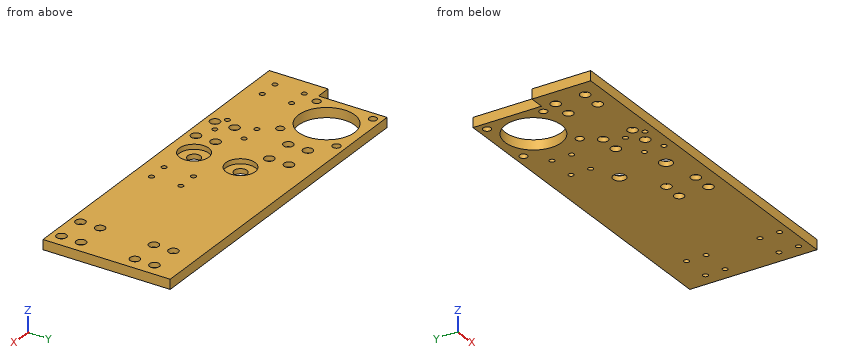
from build123d import *

# Parameters (mm, degrees)
SKETCH_1_R          = 11.5
SKETCH_1_R_2        = 1.6
SKETCH_1_R_3        = 1.05
SKETCH_1_R_4        = 2.6
EXTRUDE_1_DEPTH     = 4
SKETCH_2_R          = 2
SKETCH_2_R_2        = 6
CUT_EXTRUDE_1_DEPTH = 2
SKETCH_5_R          = 2
CUT_EXTRUDE_2_DEPTH = 2


with BuildPart() as part:
    # 草图1 → 凸台-拉伸1 (new body)
    with BuildSketch(Plane.XY):
        Polygon((0, 0), (135, 0), (135, -52), (0, -52), (-8, -52), (-8, -28), (-2, -28), (-2, 0), align=None)
        with Locations((13, -15)):
            Circle(SKETCH_1_R, mode=Mode.SUBTRACT)
        with Locations((1.5, -3.5)):
            Circle(SKETCH_1_R_2, mode=Mode.SUBTRACT)
        with Locations((24.5, -3.5)):
            Circle(SKETCH_1_R_2, mode=Mode.SUBTRACT)
        with Locations((1.5, -26.5)):
            Circle(SKETCH_1_R_2, mode=Mode.SUBTRACT)
        with Locations((24.5, -26.5)):
            Circle(SKETCH_1_R_2, mode=Mode.SUBTRACT)
        with Locations((32.5, -10)):
            Circle(SKETCH_1_R_3, mode=Mode.SUBTRACT)
        with Locations((44.5, -10)):
            Circle(SKETCH_1_R_3, mode=Mode.SUBTRACT)
        with Locations((32.5, -18)):
            Circle(SKETCH_1_R_3, mode=Mode.SUBTRACT)
        with Locations((44.5, -18)):
            Circle(SKETCH_1_R_3, mode=Mode.SUBTRACT)
        with Locations((117.5, -10)):
            Circle(SKETCH_1_R_3, mode=Mode.SUBTRACT)
        with Locations((129.5, -10)):
            Circle(SKETCH_1_R_3, mode=Mode.SUBTRACT)
        with Locations((117.5, -18)):
            Circle(SKETCH_1_R_3, mode=Mode.SUBTRACT)
        with Locations((129.5, -18)):
            Circle(SKETCH_1_R_3, mode=Mode.SUBTRACT)
        with Locations((-0.75, -33)):
            Circle(SKETCH_1_R_3, mode=Mode.SUBTRACT)
        with Locations((7.25, -33)):
            Circle(SKETCH_1_R_3, mode=Mode.SUBTRACT)
        with Locations((-0.75, -45)):
            Circle(SKETCH_1_R_3, mode=Mode.SUBTRACT)
        with Locations((7.25, -45)):
            Circle(SKETCH_1_R_3, mode=Mode.SUBTRACT)
        with Locations((29.25, -33)):
            Circle(SKETCH_1_R_3, mode=Mode.SUBTRACT)
        with Locations((37.25, -33)):
            Circle(SKETCH_1_R_3, mode=Mode.SUBTRACT)
        with Locations((37.25, -45)):
            Circle(SKETCH_1_R_3, mode=Mode.SUBTRACT)
        with Locations((29.25, -45)):
            Circle(SKETCH_1_R_3, mode=Mode.SUBTRACT)
        with Locations((32.5, -40)):
            Circle(SKETCH_1_R_3, mode=Mode.SUBTRACT)
        with Locations((44.5, -40)):
            Circle(SKETCH_1_R_3, mode=Mode.SUBTRACT)
        with Locations((32.5, -48)):
            Circle(SKETCH_1_R_3, mode=Mode.SUBTRACT)
        with Locations((44.5, -48)):
            Circle(SKETCH_1_R_3, mode=Mode.SUBTRACT)
        with Locations((117.5, -40)):
            Circle(SKETCH_1_R_3, mode=Mode.SUBTRACT)
        with Locations((129.5, -40)):
            Circle(SKETCH_1_R_3, mode=Mode.SUBTRACT)
        with Locations((117.5, -48)):
            Circle(SKETCH_1_R_3, mode=Mode.SUBTRACT)
        with Locations((129.5, -48)):
            Circle(SKETCH_1_R_3, mode=Mode.SUBTRACT)
        with Locations((55, -23)):
            Circle(SKETCH_1_R_4, mode=Mode.SUBTRACT)
        with Locations((55, -42)):
            Circle(SKETCH_1_R_4, mode=Mode.SUBTRACT)
        with Locations((77.25, -33)):
            Circle(SKETCH_1_R_3, mode=Mode.SUBTRACT)
        with Locations((77.25, -45)):
            Circle(SKETCH_1_R_3, mode=Mode.SUBTRACT)
        with Locations((69.25, -45)):
            Circle(SKETCH_1_R_3, mode=Mode.SUBTRACT)
        with Locations((69.25, -33)):
            Circle(SKETCH_1_R_3, mode=Mode.SUBTRACT)
    extrude(amount=EXTRUDE_1_DEPTH)

    # 草图2 → 切除-拉伸1 (cut)
    with BuildSketch(Plane.XY.offset(4)):
        with Locations((32.5, -10)):
            Circle(SKETCH_2_R)
        with Locations((44.5, -10)):
            Circle(SKETCH_2_R)
        with Locations((32.5, -18)):
            Circle(SKETCH_2_R)
        with Locations((44.5, -18)):
            Circle(SKETCH_2_R)
        with Locations((117.5, -10)):
            Circle(SKETCH_2_R)
        with Locations((129.5, -10)):
            Circle(SKETCH_2_R)
        with Locations((117.5, -18)):
            Circle(SKETCH_2_R)
        with Locations((129.5, -18)):
            Circle(SKETCH_2_R)
        with Locations((32.5, -40)):
            Circle(SKETCH_2_R)
        with Locations((44.5, -40)):
            Circle(SKETCH_2_R)
        with Locations((32.5, -48)):
            Circle(SKETCH_2_R)
        with Locations((44.5, -48)):
            Circle(SKETCH_2_R)
        with Locations((117.5, -40)):
            Circle(SKETCH_2_R)
        with Locations((129.5, -40)):
            Circle(SKETCH_2_R)
        with Locations((117.5, -48)):
            Circle(SKETCH_2_R)
        with Locations((55, -23)):
            Circle(SKETCH_2_R_2)
        with Locations((129.5, -48)):
            Circle(SKETCH_2_R)
        with Locations((55, -42)):
            Circle(SKETCH_2_R_2)
    extrude(amount=-CUT_EXTRUDE_1_DEPTH, mode=Mode.SUBTRACT)

    # 草图5 → 切除-拉伸2 (cut)
    with BuildSketch(Plane(origin=(0, 0, 0), x_dir=(-1, 0, 0), z_dir=(0, 0, -1))):
        with Locations((-37.25, -33)):
            Circle(SKETCH_5_R)
        with Locations((-29.25, -33)):
            Circle(SKETCH_5_R)
        with Locations((-37.25, -45)):
            Circle(SKETCH_5_R)
        with Locations((-29.25, -45)):
            Circle(SKETCH_5_R)
        with Locations((-7.25, -33)):
            Circle(SKETCH_5_R)
        with Locations((0.75, -33)):
            Circle(SKETCH_5_R)
        with Locations((-7.25, -45)):
            Circle(SKETCH_5_R)
        with Locations((0.75, -45)):
            Circle(SKETCH_5_R)
        with Locations((-69.25, -33)):
            Circle(SKETCH_5_R)
        with Locations((-69.25, -45)):
            Circle(SKETCH_5_R)
        with Locations((-77.25, -45)):
            Circle(SKETCH_5_R)
        with Locations((-77.25, -33)):
            Circle(SKETCH_5_R)
    extrude(amount=-CUT_EXTRUDE_2_DEPTH, mode=Mode.SUBTRACT)


solid = part.part
The model under review builds one solid part; all positions refer to its coordinate system, in mm. Round coordinates to 2 decimals unless told otherwise and drop trailing zeros. Loops run counter-clockwise (first coordinate to the right, second up) from the corner with the lowest first, then second, coordinate; pieces in that order, holes last. Notation, with made-up numbers: (81.5, -37) -> (123.5, -37) arc R7 ccw to (123.5, -25) -> close; hole circle Ø8 at (46, 88.25). An arc over 180 degrees is marked (long way). Write item = value, one per line. Start each with the question number.
Item 1: Take a section at A-A on x = 55. Give the boundary of the cut face in (y, z).
Item 2: Take a section at C-C on x = 16.5. Give the boundary of the cut face in (y, z), plus the area to 3 significant figures.
Item 3: To check wall thickness, follow L1, parallel to Y at x = 37.25, z = 0.7; L2, parallel to Y at x = 117.5, z = 3.15; L3, parallel to X at y = -18, z = 0.5. State the ranges of each line that lie inside material, in increasing order.
Item 4: Insertion check: pin 1 (1 mm diameter, centred on x = 75.5, y = -8, fed in from -Z); pin 2 (2 mm diameter, centred on x = 129.5, y = -17.5, fed in from +Z); pin 3 (1.7 mm diameter, centred on x = 44.5, y = -40, fed in from +Z). Each pin has a flat end and moves straight along its axis. Give the tip position at first contact, or say it passes through.
Item 5: Take a section at B-B on y = -23. Give the boundary of the cut face in (x, z).
Result:
q1.outline = (-52, 0) -> (-44.6, 0) -> (-44.6, 2) -> (-48, 2) -> (-48, 4) -> (-52, 4) -> close; (-39.4, 0) -> (-25.6, 0) -> (-25.6, 2) -> (-29, 2) -> (-29, 4) -> (-36, 4) -> (-36, 2) -> (-39.4, 2) -> close; (-20.4, 0) -> (0, 0) -> (0, 4) -> (-17, 4) -> (-17, 2) -> (-20.4, 2) -> close
q2.outline = (-52, 0) -> (-25.95, 0) -> (-25.95, 4) -> (-52, 4) -> close; (-4.05, 0) -> (0, 0) -> (0, 4) -> (-4.05, 4) -> close
q2.area = 120 mm²
q3.L1 = -52 to -47, -43 to -35, -31 to 0
q3.L2 = -52 to -50, -46 to -42, -38 to -20, -16 to -12, -8 to 0
q3.L3 = -2 to 1.9, 24.1 to 31.45, 33.55 to 43.45, 45.55 to 116.45, 118.55 to 128.45, 130.55 to 135
q4.pin_1 = 0
q4.pin_2 = 2
q4.pin_3 = through
q5.outline = (-2, 0) -> (4.74, 0) -> (4.74, 4) -> (-2, 4) -> close; (21.26, 0) -> (52.4, 0) -> (52.4, 2) -> (49, 2) -> (49, 4) -> (21.26, 4) -> close; (57.6, 0) -> (135, 0) -> (135, 4) -> (61, 4) -> (61, 2) -> (57.6, 2) -> close
